from build123d import *

# Parameters (mm, degrees)
SKETCH2_R         = 6
HUB_DEPTH         = 3
HUB_DEPTH_BACK    = 6.75
SPOKE_DEPTH       = 6.75
CIRPATTERN2_COUNT = 6


with BuildPart() as part:
    # Sketch1 → RIM (revolve)
    with BuildSketch(Plane(origin=(0, 0, 0), x_dir=(1, 0, 0), z_dir=(0, 1, 0))):
        Polygon((30.55, 6.75), (24.55, 6.75), (24.55, -6.75), (30.55, -6.75), (30.55, -5.5), (27.75, -5.5), (27.75, -3.1), (31.55, -3.1), (31.55, 3.1), (27.75, 3.1), (27.75, 5.5), (30.55, 5.5), align=None)
    revolve(axis=Axis((0, 0, 0), (0, 0, -1)))



with BuildPart() as body_2:
    # Sketch2 → HUB (new body, two sides)
    with BuildSketch(Plane.XY) as hub_sk:
        Circle(SKETCH2_R)
        with BuildLine():
            Line((-1.405555384, 1.59375), (1.405555384, 1.59375))
            ThreePointArc((1.405555384, 1.59375), (0, -2.125), (-1.405555384, 1.59375))
        make_face(mode=Mode.SUBTRACT)
    extrude(amount=HUB_DEPTH)
    extrude(hub_sk.sketch, amount=-HUB_DEPTH_BACK)


with BuildPart() as part_1:
    add(part.part)

    add(body_2.part)  # SPOKE merges body 2
    # Sketch3 → SPOKE (add)
    with BuildSketch(Plane.XY):
        with BuildLine():
            Line((-3, 5.196152423), (-2.5, 24.422377034))
            ThreePointArc((-2.5, 24.422377034), (0, 24.55), (2.5, 24.422377034))
            Line((2.5, 24.422377034), (3, 5.196152423))
            ThreePointArc((3, 5.196152423), (2.262883255, 5.556919954), (1.483432095, 5.813727653))
            Line((1.483432095, 5.813727653), (1.035788615, 23.026715831))
            ThreePointArc((1.035788615, 23.026715831), (0, 23.05), (-1.035788615, 23.026715831))
            Line((-1.035788615, 23.026715831), (-1.483432095, 5.813727653))
            ThreePointArc((-1.483432095, 5.813727653), (-2.262883255, 5.556919954), (-3, 5.196152423))
        make_face()
    spoke = extrude(amount=-SPOKE_DEPTH)

    # CirPattern2: SPOKE ×6 about axis
    cirpattern2_axis = Axis((0, 0, 0), (0, 0, 1))
    for i in range(1, CIRPATTERN2_COUNT):
        add(spoke.rotate(cirpattern2_axis, i * 360 / CIRPATTERN2_COUNT))


solid = part_1.part
Part model, mm, in its own coordinate system. A direction names the side the tool comes from. Give positions to 0.01 mm unless a question says otherwise; leave off trailing zeros.
1) Which spindle directions (+Z, -Z, +X, -X, +Y, -Y) get a long thin tool onto all of the face, cutting with end or side? Do faces 5 (the face through (-1.4, -15, 0)), 6 (the face through (-13, 25, -5.5)), 7 (the face through (11.75, -8.24, -3.33)). Say none if no direction does.
Resolved:
face 5: +Z
face 6: none
face 7: +Z, -Z
2) Two-plate mould, pull along Y, no slides. Class faces 1 (the face through (11.57, -9.85, -3.33)), 2 (the face through (12, 9, 0)), 3 (the face through (26.469, -8.335, -4.317)), 4 (the face through (0, -25, 6.75)): released by +Y, released by -Y, zero draft, split by the parting line, or undercut.
Resolved:
face 1: undercut
face 2: undercut
face 3: split by the parting line
face 4: zero draft
3) Cut at A-A on y = 21.5. State how many separate pieces and enclosed holes the cut face has, then the cut area to 3 significant figures.
Resolved:
separate pieces: 4
enclosed holes: 0
area: 264 mm2
4) Probe L1, parallel to Y at x = 0, z = -4.5 (3 decimals); L2, parallel to Y at x = 0, z = -2.5 (3 decimals); L3, parallel to X at y = 0, z = 3.5. List the from-to ranges inside material, lowest first.
Resolved:
L1: y = -27.75 to -23.05, -6 to -2.125, 1.594 to 6, 23.05 to 27.75
L2: y = -31.55 to -23.05, -6 to -2.125, 1.594 to 6, 23.05 to 31.55
L3: x = -27.75 to -24.55, 24.55 to 27.75
5) Pin check, flat tips, straight feed: pin 1 (8 mm diameter, centred on x = -12.5, z = -3.5, fed in from -Y); pin 2 (5 mm diameter, centred on x = 0.5, y = 14, fed in from +Z); pin 3 (1.4 mm diameter, centred on x = 0, z = -4, fed in from -Y). Stop position of each tip, or through.
Resolved:
pin 1: stops at y = -30.38
pin 2: stops at z = 0
pin 3: stops at y = -27.75
